Geometry: final body of the model. Coordinates: model frame, mm. A direction names the side the tool comes from. Coordinates: 2 decimals unless noted, no trailing zeros. Loops run counter-clockwise (first coordinate to the right, second up) from the corner with the lowest first, then second, coordinate; pieces in that order, holes last. Notation, with made-up numbers: M 75,62.25 L 130,62.25 A16 ccw 130,91.25 Z; hole C -36.5,14.25 d5. An arc over 180 degrees is marked long. Write item = value, one per line. Start each with the question number.
```python
from build123d import *

# Parameters (mm, degrees)
SKETCH1_R           = 8.5
BOSS_EXTRUDE1_DEPTH = 3
BOSS_EXTRUDE2_DEPTH = 3
CIRPATTERN2_COUNT   = 12
FILLET5_R           = 6
FILLET6_R           = 6
BOSS_EXTRUDE5_DEPTH = 3
SKETCH15_R          = 5
BOSS_EXTRUDE6_DEPTH = 1.9
SKETCH14_R          = 1.25
CUT_EXTRUDE7_DEPTH  = 28.730582035
SKETCH17_R          = 1.25
CUT_EXTRUDE9_DEPTH  = 28.730582035
FILLET7_R           = 2.5
BOSS_EXTRUDE7_DEPTH = 3
SKETCH20_R          = 1.25
CUT_EXTRUDE10_DEPTH = 3
FILLET8_R           = 5
FILLET9_R           = 5
FILLET10_R          = 2
FILLET11_R          = 2


# Some blends are built 0.0001 mm under size
with BuildPart() as part:
    # Sketch1 → Boss-Extrude1 (new body)
    with BuildSketch(Plane.XY):
        Circle(SKETCH1_R)
    extrude(amount=BOSS_EXTRUDE1_DEPTH)

    # Sketch3 → Boss-Extrude2 (add)
    with BuildSketch(Plane.XY.offset(3)):
        Polygon((-1.305261922, 9.914448614), (-1.509060022, 7), (1.509060022, 7), (1.305261922, 9.914448614), (0.678518537, 11), (-0.678518537, 11), align=None)
    boss_extrude2 = extrude(amount=-BOSS_EXTRUDE2_DEPTH)

    # CirPattern2: Boss-Extrude2 ×12 about axis
    cirpattern2_axis = Axis((0, 0, 0), (0, 0, 1))
    for i in range(1, CIRPATTERN2_COUNT):
        add(boss_extrude2.rotate(cirpattern2_axis, i * 360 / CIRPATTERN2_COUNT))

    # Fillet5
    # the kernel refuses this fillet: 6 mm, written as the material it takes off along each edge
    with BuildSketch(Plane(origin=(9.238795325, 3.826834324, 6.454382408), x_dir=(0.4999999999998129, 0.8660254037845467, 0), z_dir=(0, 0, -1)), Plane(origin=(1.305261922, 9.914448614, 6.454382408), x_dir=(-0.5000000000001841, 0.8660254037843323, 0), z_dir=(0, 0, -1)), Plane(origin=(-7.933533403, 6.08761429, 6.454382408), x_dir=(-1, 0, 0), z_dir=(0, 0, -1)), Plane(origin=(-9.914448614, 1.305261922, 6.454382408), x_dir=(-0.8660254037843317, -0.5000000000001852, 0), z_dir=(0, 0, -1)), Plane(origin=(-9.238795325, -3.826834324, 6.454382408), x_dir=(-0.49999999999981826, -0.8660254037845436, 0), z_dir=(0, 0, -1)), Plane(origin=(-6.08761429, -7.933533403, 6.454382408), x_dir=(0, -1, 0), z_dir=(0, 0, -1)), Plane(origin=(3.826834324, -9.238795325, 6.454382408), x_dir=(0.866025403784545, -0.49999999999981576, 0), z_dir=(0, 0, -1)), Plane(origin=(7.933533403, -6.08761429, 6.454382408), x_dir=(1, 0, 0), z_dir=(0, 0, -1)), Plane(origin=(9.914448614, -1.305261922, 6.454382408), x_dir=(0.8660254037843321, 0.5000000000001844, 0), z_dir=(0, 0, -1))) as fillet5_piece_1:
        with BuildLine():
            CenterArc((1.388315544, -5.998484909), FILLET5_R, 91.287628333, 24.712371667)
            Line((-1.241911337, -0.605720631), (-1.294515874, -0.497865346))
            Line((-1.294515874, -0.497865346), (-0.052604538, 0.107855286))
            Line((-0.052604538, 0.107855286), (0, 0.12))
            ThreePointArc((0, 0.12), (0.626743385, 0.12), (1.250790195, 0.119969698))
            Line((1.250790195, 0.119969698), (1.25348677, 0))
        make_face()
    extrude(amount=9.908764816, mode=Mode.SUBTRACT)
    with BuildSketch(Plane(origin=(6.08761429, 7.933533403, 6.454382408), x_dir=(-0.4383711467890806, -0.8987940462991654, 0), z_dir=(0, 0, -1)), Plane(origin=(-3.826834324, 9.238795325, 6.454382408), x_dir=(0.5591929034707435, -0.8290375725550441, 0), z_dir=(0, 0, -1)), Plane(origin=(-1.305261922, -9.914448614, 6.454382408), x_dir=(-0.06975647374412178, 0.9975640502598244, 0), z_dir=(0, 0, -1))) as fillet5_piece_2:
        with BuildLine():
            CenterArc((1.381752963, 6), FILLET5_R, 245.287628333, 24.712371667)
            Line((-1.126626446, 0.549492433), (-1.176794034, 0.440482282))
            ThreePointArc((-1.176794034, 0.440482282), (-0.615917761, 0.166890931), (-0.052604538, -0.107855286))
            Line((-0.052604538, -0.107855286), (0, -0.12))
            Line((0, -0.12), (1.381752963, -0.12))
            Line((1.381752963, -0.12), (1.381752963, 0))
        make_face()
    extrude(amount=9.908764816, mode=Mode.SUBTRACT)

    # Fillet6
    # the kernel refuses this fillet: 6 mm, written as the material it takes off along each edge
    with BuildSketch(Plane(origin=(7.933533403, 6.08761429, 6.454382408), x_dir=(-0.8987940462991681, -0.4383711467890748, 0), z_dir=(0, 0, -1)), Plane(origin=(3.826834324, 9.238795325, 6.454382408), x_dir=(-0.5591929034707512, -0.8290375725550386, 0), z_dir=(0, 0, -1)), Plane(origin=(-1.305261922, 9.914448614, 6.454382408), x_dir=(-0.06975647374412959, -0.9975640502598239, 0), z_dir=(0, 0, -1)), Plane(origin=(-6.08761429, 7.933533403, 6.454382408), x_dir=(0.43837114678907496, -0.8987940462991681, 0), z_dir=(0, 0, -1)), Plane(origin=(-9.238795325, 3.826834324, 6.454382408), x_dir=(0.8290375725550394, -0.5591929034707502, 0), z_dir=(0, 0, -1)), Plane(origin=(-9.914448614, -1.305261922, 6.454382408), x_dir=(0.9975640502598241, -0.06975647374412908, 0), z_dir=(0, 0, -1)), Plane(origin=(-7.933533403, -6.08761429, 6.454382408), x_dir=(0.8987940462991686, 0.4383711467890744, 0), z_dir=(0, 0, -1)), Plane(origin=(-3.826834324, -9.238795325, 6.454382408), x_dir=(0.559192903470749, 0.8290375725550401, 0), z_dir=(0, 0, -1)), Plane(origin=(1.305261922, -9.914448614, 6.454382408), x_dir=(0.06975647374412973, 0.9975640502598241, 0), z_dir=(0, 0, -1)), Plane(origin=(6.08761429, -7.933533403, 6.454382408), x_dir=(-0.4383711467890742, 0.8987940462991686, 0), z_dir=(0, 0, -1)), Plane(origin=(9.238795325, -3.826834324, 6.454382408), x_dir=(-0.8290375725550386, 0.5591929034707512, 0), z_dir=(0, 0, -1)), Plane(origin=(9.914448614, 1.305261922, 6.454382408), x_dir=(-0.9975640502598239, 0.06975647374412945, 0), z_dir=(0, 0, -1))) as fillet6_piece_1:
        with BuildLine():
            CenterArc((1.381752963, -6), FILLET6_R, 90, 24.712371667)
            Line((-1.126626446, -0.549492433), (-1.176794034, -0.440482282))
            ThreePointArc((-1.176794034, -0.440482282), (-0.615917761, -0.166890931), (-0.052604538, 0.107855286))
            Line((-0.052604538, 0.107855286), (0, 0.12))
            Line((0, 0.12), (1.381752963, 0.12))
            Line((1.381752963, 0.12), (1.381752963, 0))
        make_face()
    extrude(amount=9.908764816, mode=Mode.SUBTRACT)

    # Sketch12 → Boss-Extrude5 (add)
    with BuildSketch(Plane(origin=(0, 0, 0), x_dir=(-1, 0, 0), z_dir=(0, 0, -1))):
        Polygon((1.535905814, 15.391336798), (-4.226547881, -6.114433171), (0.60308125, -7.408528397), (9.014700216, 23.984060958), (4.185071084, 25.278156183), align=None)
    extrude(amount=-BOSS_EXTRUDE5_DEPTH)

    # Sketch15 → Boss-Extrude6 (add)
    with BuildSketch(Plane(origin=(0, 0, 0), x_dir=(-1, 0, 0), z_dir=(0, 0, -1))):
        Circle(SKETCH15_R)
    extrude(amount=-BOSS_EXTRUDE6_DEPTH)

    # Sketch14 → Cut-Extrude7 (cut, through all)
    with BuildSketch(Plane(origin=(0, 0, 0), x_dir=(-1, 0, 0), z_dir=(0, 0, -1))):
        Circle(SKETCH14_R)
    extrude(amount=-CUT_EXTRUDE7_DEPTH, mode=Mode.SUBTRACT)

    # Sketch17 → Cut-Extrude9 (cut, through all)
    with BuildSketch(Plane.XY.offset(3)):
        with Locations((-5.952838037, 22.216294005)):
            Circle(SKETCH17_R)
    extrude(amount=-CUT_EXTRUDE9_DEPTH, mode=Mode.SUBTRACT)

    # Fillet7
    fillet7_edges = [part.edges().sort_by_distance(p)[0] for p in [
        (-9.014700216, 23.984060958, 1.5),
        (-4.185071084, 25.278156183, 1.5),
    ]]
    fillet(fillet7_edges, radius=FILLET7_R - 0.0001)  # a hair under: the kernel refuses the full size

    # Sketch19 → Boss-Extrude7 (add)
    with BuildSketch(Plane.XY.offset(3)):
        Polygon((-6.59988565, 24.63110857), (-12.395440608, 23.0781943), (-11.101345382, 18.248565168), (0.489764533, 21.35439371), (-0.804330692, 26.184022841), align=None)
    extrude(amount=-BOSS_EXTRUDE7_DEPTH)

    # Sketch20 → Cut-Extrude10 (cut)
    with BuildSketch(Plane.XY.offset(3)):
        with Locations((-9.333578429, 21.310427347)):
            Circle(SKETCH20_R)
        with Locations((-2.572097645, 23.122160663)):
            Circle(SKETCH20_R)
    extrude(amount=-CUT_EXTRUDE10_DEPTH, mode=Mode.SUBTRACT)

    # Fillet8
    # the kernel refuses this fillet: 5 mm, written as the material it adds along each edge
    with BuildSketch(Plane(origin=(-7.72060499, 19.154431826, 0), x_dir=(-0.9659258262890523, -0.25881904510258064, 0), z_dir=(0, 0, 1))) as fillet8_piece_1:
        with BuildLine():
            CenterArc((5, 4.769696007), FILLET8_R, 180, 72.542396876)
            Line((0, 4.769696007), (-0.1, 4.769696007))
            Line((-0.1, 4.769696007), (-0.1, 0))
            Line((-0.1, 0), (0, -0.1))
            ThreePointArc((0, -0.1), (1.75, -0.1), (3.47, -0.09539392))
            Line((3.47, -0.09539392), (3.5, 0))
        make_face()
    extrude(amount=3)

    # Fillet9
    # the kernel refuses this fillet: 5 mm, written as the material it adds along each edge
    with BuildSketch(Plane(origin=(-2.890975859, 20.448527052, 3), x_dir=(0.9659258262890524, 0.25881904510257997, 0), z_dir=(0, 0, -1))) as fillet9_piece_1:
        with BuildLine():
            CenterArc((5, 4.769696007), FILLET9_R, 180, 72.542396876)
            Line((0, 4.769696007), (-0.1, 4.769696007))
            Line((-0.1, 4.769696007), (-0.1, 0))
            Line((-0.1, 0), (0, -0.1))
            ThreePointArc((0, -0.1), (1.75, -0.1), (3.47, -0.09539392))
            Line((3.47, -0.09539392), (3.5, 0))
        make_face()
    extrude(amount=3)

    # Fillet10
    fillet10_edges = [part.edges().sort_by_distance(p)[0] for p in [
        (-0.804330692, 26.184022841, 1.5),
    ]]
    fillet(fillet10_edges, radius=FILLET10_R)

    # Fillet11
    fillet11_edges = [part.edges().sort_by_distance(p)[0] for p in [
        (-12.395440608, 23.0781943, 1.5),
    ]]
    fillet(fillet11_edges, radius=FILLET11_R)


solid = part.part
```
Item 1: Reachability of faces 5 (the cylindrical face through (-7.924, 5.924, 1.521)), 6 (the cylindrical face through (9.067, -3.874, 1.521)), 7 (the cylindrical face through (-5.924, -7.924, 1.521)) from +Z, -Z, +X, -X, +Y, -Y: full face, straight path, thin tool, end or side. Return the list, or none.
Item 2: Section query A-A (y = 0). Return the cut outline in (x, z).
Item 3: Pull-direction query (X, two-part tool) for faces 1 (the cylindrical face through (2.211, 8.207, 1.479)), 2 (the cylindrical face through (-2.84, 21.9, 1.52)), 3 (the cylindrical face through (-9.09, -3.9, 1.52)), 4 (the flat face through (0, -11, 2)); classes: released by +X, released by -X, zero draft, split by the parting line, or undercut.
Item 4: First-contact query: pin 1 (1.5 mm diameter, centred on y = 0.5, z = 1.5, fed in from -X); pin 2 (1 mm diameter, centred on y = 3.5, z = 1.5, fed in from +X); pin 3 (4 mm diameter, centred on x = -9.33, y = 21.31, fed in from -Z); pin 4 (1.5 mm diameter, centred on y = 18.5, z = 1.5, fed in from -X). Flat tips, straight axial feed; report the tip coordinate or a pass-through.
Item 5: Section query C-C (z = 1.85). Count the separate pieces of the cut face and the enclosed holes in it, plus the area to 3 significant figures.
Item 6: Section query B-B (x = -7.5). Return the cut outline in (y, z), plus the area to 3 significant figures.
Item 7: Line query: line 1 (X direction, y = 5.5, z = 1.25); line 2 (Y direction, x = -8.5, z = 0.9); line 3 (Y direction, x = 6.5, z = 1.75). Output: solid intervals per line, ascending. Write a range as from..to.
Item 8: Section query D-D (y = 19.5). Return the cut outline in (x, z), plus the area to 3 significant figures.
Verdict:
q1.face_5 = +Z, -Z
q1.face_6 = +Z, -Z, +X
q1.face_7 = +Z, -Z, -X
q2.outline = M -11,0 L -1.25,0 L -1.25,3 L -11,3 Z; M 1.25,0 L 11,0 L 11,3 L 1.25,3 Z
q3.face_1 = undercut
q3.face_2 = undercut
q3.face_3 = released by -X
q3.face_4 = zero draft
q4.pin_1 = -11
q4.pin_2 = 9.18
q4.pin_3 = 0
q4.pin_4 = -11.37
q5.separate_pieces = 1
q5.enclosed_holes = 3
q5.area = 404 mm2
q6.outline = M -5.81,0 L 5.81,0 L 5.81,3 L -5.81,3 Z; M 16.48,0 L 24.39,0 L 24.39,3 L 16.48,3 Z
q6.area = 58.6 mm2
q7.line_1 = -9.53..-6.73, -6.48..6.48, 6.73..9.53
q7.line_2 = -6.03..-3.35, -1.4..1.4, 3.35..6.03, 17.38..20.38, 22.24..24.12
q7.line_3 = -5.48..5.48
q8.outline = M -11.44,0 L -1.23,0 L -1.23,3 L -11.44,3 Z
q8.area = 30.6 mm2
